Part model, mm, in its own coordinate system. A direction names the side the tool comes from. Round coordinates to 2 decimals unless told otherwise and drop trailing zeros. Write each loop counter-clockwise with the first axis right and the second up, starting at its lowest first coordinate (ties: lowest second). Pieces come first, ordered by that corner, then holes. Notation, with made-up numbers: (-37.5, -3) -> (-21.5, -3) arc R8 cw to (-21.5, 3) -> close; hole circle Ø6 at (40, 11). An arc over 180 degrees is marked (long way). Return JSON: item names as keys, results as strings. Group by question number.
Autodesk Inventor part; units mm, degrees
ref_plane "YZ Plane" through (0, 0, 0) normal (1, 0, 0) x (0, 1, 0)
ref_plane "XZ Plane" through (0, 0, 0) normal (0, 1, 0) x (-1, 0, 0)
ref_plane "XY Plane" through (0, 0, 0) normal (0, 0, 1) x (1, 0, 0)
sketch "Sketch1" plane through (0, 0, 0) normal (0, 0, 1) x (1, 0, 0)
  line L0 (0, 0) -> (3.5719, 0) construction
  line L1 (1.905, 7.5269) -> (1.905, 0)
  line L2 (1.905, 0) -> (3.5719, 0)
  line L3 (0, 0) -> (0, 5.4125) construction
  line L4 (3.5719, 0) -> (2.6587, 2.509)
  line L5 (2.6587, 2.509) -> (3.5719, 2.509)
  line L6 (3.5719, 2.509) -> (2.6587, 5.0179)
  line L7 (2.6587, 5.0179) -> (3.5719, 5.0179)
  line L8 (3.5719, 5.0179) -> (2.6587, 7.5269)
  line L9 (2.6587, 7.5269) -> (1.905, 7.5269)
  point P0 (2.0609, 0)
  dimension "d0" = 3.5719
  dimension "d4" = 1.905
  dimension "d9" = 70
  dimension "d12" = 70
revolve "Revolution1" add sketch "Sketch1" angle 360 about axis through (0, 0, 0) along (0, 1, 0)
sketch "Sketch2" plane through (0, 0, 0) normal (0, -1, 0) x (1, 0, 0)
  circle A0 centre (0, 0) radius 5.08
  dimension "d5" = 10.16
extrude "Extrusion1" add sketch "Sketch2" along normal blind 3.175
sketch "Sketch4" plane through (0, -3.175, 0) normal (0, -1, 0) x (1, 0, 0)
  circle A0 centre (0, 0) radius 1.905
  circle A1 centre (0, -1.016) radius 0.762
  circle A2 centre (0.8799, 0.508) radius 0.762
  circle A3 centre (-0.8799, 0.508) radius 0.762
  dimension "d50" = 1.524
  dimension "d51" = 0.127
  dimension "d54" = 360
extrude "Extrusion3" cut sketch "Sketch4" against normal through all contours A1 | A2 | A3
properties part number "Hose Barb_3DPrint"
Item 1: Flat gauge pins, fed straight in: P1, Ø4, axis at x = 3.5, y = 1, coming from the -Z side; P2, Ø5, axis at y = 5.5, z = -3, coming from the -X side; P3, Ø6, axis at x = -4, y = 0.5, coming from the -Z side. Where does each tip first touch, or does it go through?
Item 2: Wall check: L1, parallel to Z at x = 0, y = -1.4; L2, parallel to Y at x = -4.25, z = 0.75 (3 decimals); L3, parallel to X at y = -0.25, z = 0.25. Give the ranges that are in metal, low to high.
Item 3: Cut at B-B (y = -0.75). Write the cut outline in (x, z), then the cut area to 3 significant figures.
Item 4: Which spindle directions (+Z, -Z, +X, -X, +Y, -Y) get a long thin tool onto all of the face, cutting with end or side? Do faces 4 (the face through (0, 2.509, -3)), 5 (the face through (2.2, 0, -3.3)), 6 (the face through (-2, 7.527, -1)). Say none if no direction does.
Item 5: Cut at D-D (x = 0.5). State how many separate pieces and enclosed holes the cut face has, then the cut area to 3 significant figures.
Item 6: Cut at C-C (y = 3.5). Write the cut outline in (x, z) (3 decimals).
Item 7: Cut at A-A (z = 0). Write the cut outline in (x, y) (3 decimals), then the cut area to 3 significant figures.
Item 8: Two-plate mould, pull along Y, no slides. Class faces 1 (the face through (-0.41, 3.71, -1.86)), 2 (the face through (0, 0, 0)), 3 (the face through (0, 5.018, -3)): released by +Y, released by -Y, zero draft, split by the parting line, or undercut.
Checks:
{
 "1": {"P1": "stops at z = -4.76", "P2": "stops at x = -3.53", "P3": "stops at z = -4.97"},
 "2": {"L1": "z = -5.08 to -1.78, -0.25 to 5.08", "L2": "y = -3.175 to 0", "L3": "x = -5.07 to -1.6, -0.16 to 0.16, 1.6 to 5.07"},
 "3": {"outline": "circle Ø10.16 at (0, 0); hole circle Ø1.52 at (-0.88, 0.51); hole circle Ø1.52 at (0, -1.02); hole circle Ø1.52 at (0.88, 0.51)", "area": "75.6 mm2"},
 "4": {"face 4": "none", "face 5": "+Y", "face 6": "+Z, -Z, +X, -X, +Y"},
 "5": {"separate pieces": "3", "enclosed holes": "0", "area": "42.9 mm2"},
 "6": {"outline": "circle Ø6.422 at (0, 0); hole circle Ø3.81 at (0, 0)"},
 "7": {"outline": "(-5.08, -3.175) -> (-1.448, -3.175) -> (-1.448, 0) -> (-1.905, 0) -> (-1.905, 7.527) -> (-2.659, 7.527) -> (-3.572, 5.018) -> (-2.659, 5.018) -> (-3.572, 2.509) -> (-2.659, 2.509) -> (-3.572, 0) -> (-5.08, 0) -> close; (-0.312, -3.175) -> (0.312, -3.175) -> (0.312, 0) -> (-0.312, 0) -> close; (1.448, -3.175) -> (5.08, -3.175) -> (5.08, 0) -> (3.572, 0) -> (2.659, 2.509) -> (3.572, 2.509) -> (2.659, 5.018) -> (3.572, 5.018) -> (2.659, 7.527) -> (1.905, 7.527) -> (1.905, 0) -> (1.448, 0) -> close", "area": "43.3 mm2"},
 "8": {"face 1": "zero draft", "face 2": "released by +Y", "face 3": "undercut"}
}
